Autodesk Inventor part; units mm, degrees
ref_plane "YZ Plane" through (0, 0, 0) normal (1, 0, 0) x (0, 1, 0)
ref_plane "XZ Plane" through (0, 0, 0) normal (0, 1, 0) x (-1, 0, 0)
ref_plane "XY Plane" through (0, 0, 0) normal (0, 0, 1) x (1, 0, 0)
sketch "Sketch1" plane through (0, 0, 0) normal (0, 0, 1) x (1, 0, 0)
  line L0 (-46.101, -41.8465) -> (-39.116, -41.8465)
  line L1 (46.101, -41.8465) -> (46.101, -34.8721)
  line L2 (46.101, 41.8465) -> (-46.101, 41.8465)
  line L3 (-46.101, 41.8465) -> (-46.101, 34.8721)
  line L4 (-46.101, -41.8465) -> (46.101, 41.8465) construction
  line L5 (46.101, -41.8465) -> (-46.101, 41.8465) construction
  line L6 (-40.005, 41.8465) -> (-40.005, 34.8721) construction
  line L7 (40.005, -41.8465) -> (40.005, -34.8721)
  line L8 (-40.005, -29.4005) -> (-33.3375, -29.4005) construction
  line L9 (-40.005, -35.4965) -> (-33.3375, -35.4965) construction
  line L10 (-33.3375, -29.4005) -> (-33.3375, -35.4965) construction
  line L11 (-13.335, -29.4005) -> (-13.335, -35.4965) construction
  line L12 (-33.3375, -29.4005) -> (-13.335, -29.4005) construction
  line L13 (-13.335, -29.4005) -> (-4.0005, -29.4005) construction
  line L14 (-13.335, -35.4965) -> (-4.0005, -35.4965) construction
  line L15 (-33.3375, -35.4965) -> (-13.335, -35.4965) construction
  line L16 (-64.5414, 0) -> (64.5414, 0) construction
  line L17 (-46.101, 34.8721) -> (-40.005, 34.8721) construction
  line L18 (-46.101, 27.8977) -> (-40.005, 27.8977) construction
  line L19 (40.005, 34.8721) -> (46.101, 34.8721)
  line L20 (-46.101, 34.8721) -> (-46.101, 34.8086)
  line L21 (-46.101, 27.8977) -> (-46.101, 10.3981)
  line L22 (-40.005, 34.8721) -> (-40.005, 27.8977) construction
  line L23 (-40.005, 27.8977) -> (-40.005, 10.4616) construction
  line L24 (46.101, 34.8721) -> (46.101, 41.8465)
  line L25 (40.005, 34.8721) -> (40.005, 41.8465)
  line L26 (-33.274, -35.4648) -> (-13.3985, -35.4648)
  line L27 (-13.3985, -35.4648) -> (-13.3985, -29.4323)
  line L28 (-13.3985, -29.4323) -> (-33.274, -29.4323)
  line L29 (-33.274, -29.4323) -> (-33.274, -35.4648)
  line L30 (-33.274, -35.4648) -> (-13.3985, -29.4323) construction
  line L31 (-13.3985, -35.4648) -> (-33.274, -29.4323) construction
  line L32 (-23.3362, -32.4485) -> (-23.3362, -29.4005) construction
  line L33 (-23.3362, -32.4485) -> (-13.335, -32.4485) construction
  line L34 (-46.101, 34.8086) -> (-40.0367, 34.8086)
  line L35 (-40.0367, 34.8086) -> (-40.0367, 27.9612)
  line L36 (-40.0367, 27.9612) -> (-46.101, 27.9612)
  line L37 (-40.0367, 31.3849) -> (-40.005, 31.3849) construction
  line L38 (-46.101, 34.8086) -> (-46.101, 27.9612)
  line L39 (-46.101, 27.9612) -> (-46.101, 27.8977)
  arc A0 (39.116, -41.8465) -> (-39.116, -41.8465) centre (0, -215.2904) ccw
  line L40 (0, 93.2739) -> (0, -266.7178) construction
  line L41 (-39.116, -41.8465) -> (39.116, -41.8465)
  line L42 (39.116, -41.8465) -> (40.005, -41.8465)
  line L43 (-4.0005, -29.4005) -> (-4.0005, -35.4965) construction
  line L44 (4.0005, -29.4005) -> (4.0005, -35.4965) construction
  line L45 (13.335, -29.4005) -> (13.335, -35.4965) construction
  line L46 (33.3375, -29.4005) -> (33.3375, -35.4965) construction
  line L47 (-3.937, -35.4648) -> (3.937, -35.4648)
  line L48 (3.937, -35.4648) -> (3.937, -29.4323)
  line L49 (3.937, -29.4323) -> (-3.937, -29.4323)
  line L50 (-3.937, -29.4323) -> (-3.937, -35.4648)
  line L51 (-3.937, -35.4648) -> (3.937, -29.4323) construction
  line L52 (3.937, -35.4648) -> (-3.937, -29.4323) construction
  line L53 (13.3985, -35.4648) -> (33.274, -35.4648)
  line L54 (33.274, -35.4648) -> (33.274, -29.4323)
  line L55 (33.274, -29.4323) -> (13.3985, -29.4323)
  line L56 (13.3985, -29.4323) -> (13.3985, -35.4648)
  line L57 (13.3985, -35.4648) -> (33.274, -29.4323) construction
  line L58 (33.274, -35.4648) -> (13.3985, -29.4323) construction
  line L59 (-4.0005, -35.4965) -> (4.0005, -35.4965) construction
  line L60 (4.0005, -35.4965) -> (13.335, -35.4965) construction
  line L61 (4.0005, -29.4005) -> (13.335, -29.4005) construction
  line L62 (-4.0005, -29.4005) -> (4.0005, -29.4005) construction
  line L63 (13.335, -29.4005) -> (33.3375, -29.4005) construction
  line L64 (33.3375, -29.4005) -> (40.005, -29.4005) construction
  line L65 (33.3375, -35.4965) -> (40.005, -35.4965) construction
  line L66 (13.335, -35.4965) -> (33.3375, -35.4965) construction
  line L67 (23.3362, -29.4005) -> (23.3362, -32.4485) construction
  line L68 (-46.101, 10.4616) -> (-40.005, 10.4616) construction
  line L69 (-46.101, 3.4872) -> (-40.005, 3.4872) construction
  line L70 (-46.101, -3.4872) -> (-40.005, -3.4872) construction
  line L71 (-46.101, -10.4616) -> (-40.005, -10.4616) construction
  line L72 (-46.101, -27.8977) -> (-40.005, -27.8977) construction
  line L73 (-46.101, -34.8721) -> (-40.005, -34.8721) construction
  line L74 (-46.101, 10.3981) -> (-40.0367, 10.3981)
  line L75 (-40.0367, 10.3981) -> (-40.0367, 3.5507)
  line L76 (-40.0367, 3.5507) -> (-46.101, 3.5507)
  line L77 (-46.101, -3.5507) -> (-40.0367, -3.5507)
  line L78 (-40.0367, -3.5507) -> (-40.0367, -10.3981)
  line L79 (-40.0367, -10.3981) -> (-46.101, -10.3981)
  line L80 (-46.101, -27.9612) -> (-40.0367, -27.9612)
  line L81 (-40.0367, -27.9612) -> (-40.0367, -34.8086)
  line L82 (-40.0367, -34.8086) -> (-46.101, -34.8086)
  line L83 (-40.005, 10.4616) -> (-40.005, 3.4872) construction
  line L84 (-40.005, 3.4872) -> (-40.005, -3.4872) construction
  line L85 (-40.005, -3.4872) -> (-40.005, -10.4616) construction
  line L86 (-40.005, -10.4616) -> (-40.005, -27.8977) construction
  line L87 (-40.005, -34.8721) -> (-40.005, -41.8465) construction
  line L88 (-40.005, -27.8977) -> (-40.005, -34.8721) construction
  line L89 (-40.0367, -31.3849) -> (-40.005, -31.3849) construction
  line L90 (-40.0367, -6.9744) -> (-40.005, -6.9744) construction
  line L91 (-40.0367, 6.9744) -> (-40.005, 6.9744) construction
  line L92 (-46.101, 10.3981) -> (-46.101, 3.5507)
  line L93 (-46.101, 3.5507) -> (-46.101, -3.5507)
  line L94 (-46.101, -10.3981) -> (-46.101, -27.9612)
  line L95 (-46.101, -3.5507) -> (-46.101, -10.3981)
  line L96 (-46.101, -34.8086) -> (-46.101, -41.8465)
  line L97 (-46.101, -27.9612) -> (-46.101, -34.8086)
  line L98 (46.101, 27.8977) -> (40.005, 27.8977)
  line L99 (40.005, 3.4872) -> (46.101, 3.4872)
  line L100 (40.005, -3.4872) -> (46.101, -3.4872)
  line L101 (40.005, -10.4616) -> (46.101, -10.4616)
  line L102 (40.005, -27.8977) -> (46.101, -27.8977)
  line L103 (40.005, 10.4616) -> (46.101, 10.4616)
  line L104 (40.005, -34.8721) -> (46.101, -34.8721)
  line L105 (40.005, -27.8977) -> (40.005, -10.4616)
  line L106 (40.005, -34.8721) -> (40.005, -27.8977) construction
  line L107 (40.005, -10.4616) -> (40.005, -3.4872) construction
  line L108 (40.005, -3.4872) -> (40.005, 3.4872)
  line L109 (40.005, 3.4872) -> (40.005, 10.4616) construction
  line L110 (40.005, 10.4616) -> (40.005, 27.8977)
  line L111 (40.005, 27.8977) -> (40.005, 34.8721) construction
  line L112 (40.005, -41.8465) -> (46.101, -41.8465)
  line L113 (46.101, -34.8721) -> (46.101, -27.8977)
  line L114 (46.101, -27.8977) -> (46.101, -10.4616)
  line L115 (46.101, -10.4616) -> (46.101, -3.4872)
  line L116 (46.101, -3.4872) -> (46.101, 3.4872)
  line L117 (46.101, 3.4872) -> (46.101, 10.4616)
  line L118 (46.101, 10.4616) -> (46.101, 27.8977)
  line L119 (46.101, 27.8977) -> (46.101, 34.8721)
  point P0 (0, 0)
  point P1 (0, -32.4485)
  dimension "d1" = 6.096
  dimension "d3" = 6.096
  dimension "d4" = 6.35
  dimension "d5" = 20.0025
  dimension "d6" = 13.335
  dimension "d9" = 83.693
  dimension "d10" = 6.9744
  dimension "d11" = 71.247
  dimension "d12" = 6.9744
  dimension "d32" = 6.0325
  dimension "d33" = 19.8755
  dimension "d34" = 6.8474
  dimension "d36" = 6.0643
  dimension "d38" = 6.985
  dimension "d39" = 177.8
  dimension "d40" = 8.001
  dimension "d41" = 4.0005
  dimension "d42" = 20.0025
  dimension "d43" = 7.874
  dimension "d44" = 19.8755
  dimension "d45" = 13.335
  dimension "d46" = 6.9744
  dimension "d47" = 6.9744
  dimension "d48" = 6.8474
  dimension "d49" = 6.8474
  dimension "d50" = 6.8474
  dimension "d51" = 80.01
  dimension "d52" = 6.096
extrude "Extrusion1" add sketch "Sketch1" along normal blind 6.096 contours L96 L82 L81 L80 L94 L79 L78 L77 L93 L76 L75 L74 L21 L39 L36 L35 L34 L20 L3 L2 L25 L19 L119 L98 L110 L103 L117 L99 L108 L100 L115 L101 L105 L102 L113 L104 L7 L42 A0 L0 | L38 L34 L35 L36 | L19 L25 L2 L24 | L29 L28 L27 L26 | L50 L49 L48 L47 | L56 L55 L54 L53
extrude "Extrusion2" cut sketch "Sketch1" along normal blind 6.096 contours L19 L25 L2 L24
extrude "Extrusion3" cut sketch "Sketch1" along normal blind 6.096 contours L38 L34 L35 L36
extrude "Extrusion4" cut sketch "Sketch1" along normal blind 6.096 contours L29 L28 L27 L26 | L50 L49 L48 L47 | L56 L55 L54 L53
fillet "Fillet1" [suppressed]
fillet "Fillet2" [suppressed]
equation "\"d1\" = woodThickness"
equation "\"d3\" = woodThickness"
equation "\"d5\" = toothLength"
equation "\"d10\" = 0.0833333 * d9"
equation "\"d11\" = glassHeight - lip"
equation "\"d12\" = d10"
equation "\"d32\" = d1 - lasorTol"
equation "\"d33\" = d5 - 2 * lasorTol"
equation "\"d34\" = d12 - 2 * lasorTol"
equation "\"d36\" = d3 - 0.5 * lasorTol"
equation "\"d40\" = 0.4 * toothLength"
equation "\"d41\" = 0.5 * d40"
equation "\"d42\" = d5"
equation "\"d43\" = d40 - 2 * lasorTol"
equation "\"d44\" = d42 - 2 * lasorTol"
equation "\"d45\" = d6"
equation "\"d46\" = d12"
equation "\"d47\" = d10"
equation "\"d48\" = d34"
equation "\"d49\" = d34"
equation "\"d50\" = d34"
equation "\"d51\" = baseLength"
equation "\"d52\" = woodThickness"
equation "\"d13\" = woodThickness"
equation "\"d15\" = woodThickness"
equation "\"d17\" = woodThickness"
equation "\"d19\" = woodThickness"
properties part number "CandleHolder-2" material "Wood (Birch)"
CAD build for the part. Positions are in the model's coordinates, mm. A direction names the side the tool comes from. Round coordinates to 2 decimals unless told otherwise and drop trailing zeros. Order: outer loops, then holes, each group sorted by start corner. A loop starts at its lowest first (then second) coordinate and runs counter-clockwise, first axis right, second up. Notation, with made-up numbers: (27, -34.75) - (51, -34.75) arc R28 cw to (51, -4.75) - close; hole circle Ø9 at (51.25, 20). An arc over 180 degrees is marked (long way). Use CSV: the item, a comma, the result in double quotes. Start each with the question number.
1) Saw through at B-B (x = -24.5). List the corners of the cut face in (y, z), and give its area (3 significant figures).
2) Pin check, flat tips, straight feed: pin 1 Ø1.8 at (y, z) = (-32.5, 3) entering from -X; pin 2 Ø3 at (x, z) = (44.5, 1.5) entering from -Y; pin 3 Ø3 at (x, z) = (1.5, 4.5) entering from -Y. Stop position of each tip, or through.
3) Two-plate mould, pull along X, no slides. Class faces 1 (the flat face through (3.937, -32, 3)), 2 (the flat face through (-46.101, 19, 3)), 3 (the flat face through (-1, 1, 6.096)): pulls with the +X half, pulls with the -X half, needs draft (parallel to the pull), parting line crosses it, or undercut.
4) Tool access for faces 4 (the flat face through (43, 27.898, 3)), 5 (the flat face through (40.005, -38, 3)), 6 (the flat face through (23, -29.432, 3)), 7 (the flat face through (-43, 3.551, 3)): list every direction of +Z, -Z, +X, -X, +Y, -Y with a clear straight run to the whole face (end or side of a thin tool).
5) Saw through at D-D (y = 5.5). List the corners of the cut face in (x, z).
6) Saw through at A-A (y = -31.5). List the corners of the cut face in (x, z), and give its area (3 significant figures).
7) Saw through at C-C (z = 1.75). Count the separate pieces of the cut face and the enclosed holes in it, and give its area (3 significant figures).
8) Wall check: L1, parallel to X at y = -30.5, z = 4.75; L2, parallel to Y at x = 2, z = 1.25; L3, parallel to Y at x = 40.5, z = 5.75. Give the ranges that are in metal, low to high. Write a range as [from, to].
Values follow:
1,outline,"(-39.19, 0) - (-35.46, 0) - (-35.46, 6.1) - (-39.19, 6.1) - close; (-29.43, 0) - (41.85, 0) - (41.85, 6.1) - (-29.43, 6.1) - close"
1,area,"457 mm2"
2,pin 1,"stops at x = -40.04"
2,pin 2,"stops at y = -34.87"
2,pin 3,"stops at y = -37.52"
3,face 1,"undercut"
3,face 2,"pulls with the -X half"
3,face 3,"needs draft"
4,face 4,"+Z, -Z, +X"
4,face 5,"+Z, -Z, +X, -Y"
4,face 6,"+Z, -Z"
4,face 7,"+Z, -Z, -X"
5,outline,"(-40.04, 0) - (46.1, 0) - (46.1, 6.1) - (-40.04, 6.1) - close"
6,outline,"(-40.04, 0) - (-33.27, 0) - (-33.27, 6.1) - (-40.04, 6.1) - close; (-13.4, 0) - (-3.94, 0) - (-3.94, 6.1) - (-13.4, 6.1) - close; (3.94, 0) - (13.4, 0) - (13.4, 6.1) - (3.94, 6.1) - close; (33.27, 0) - (46.1, 0) - (46.1, 6.1) - (33.27, 6.1) - close"
6,area,"235 mm2"
7,separate pieces,"1"
7,enclosed holes,"3"
7,area,"6,700 mm2"
8,L1,"x = [-40.04, -33.27], [-13.4, -3.94], [3.94, 13.4], [33.27, 46.1]"
8,L2,"y = [-37.5, -35.46], [-29.43, 41.85]"
8,L3,"y = [-34.87, -27.9], [-10.46, -3.49], [3.49, 10.46], [27.9, 34.87]"
